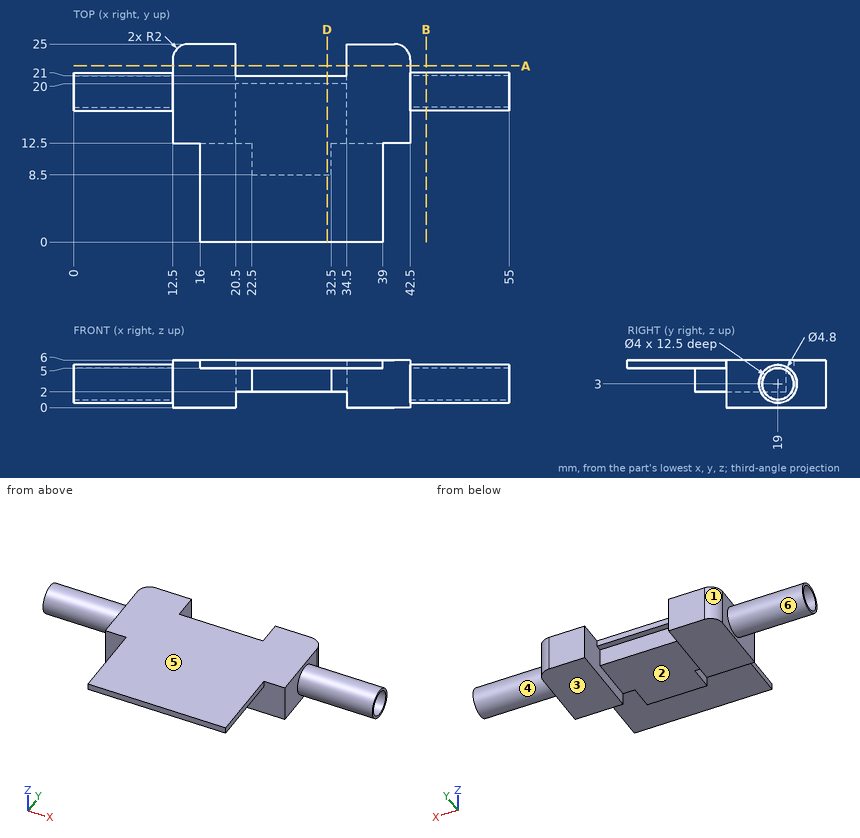
Verification items for this drawing (mm, ordinates from the low corner). A direction names the side the tool comes from. Round coordinates to 2 decimals unless told otherwise and drop trailing zeros. Loops run counter-clockwise (first coordinate to the right, second up) from the corner with the lowest first, then second, coordinate; pieces in that order, holes last. Notation, with made-up numbers: (33.25, 31.25) -> (60.25, 31.25) arc R21 cw to (60.25, 36.25) -> close; hole circle Ø7 at (-12, 40.5). An arc over 180 degrees is marked (long way). Write item = value, one per line. Start each with the question number.
1) Thickness scan on probe 1 along Y at (x, z) = (52.75, 3); probe 2 along Y at (x, z) = (22, 4.9); probe 3 along X at (y, z) = (15, 3.05). Record the ranges inside material, lowest first.
2) Release check for a two-part mould opening along X. For the marked faces 1, 2 and 3 record: released by +X, released by -X, zero draft, split by the parting line, or undercut.
3) Sectioned sample at B-B, the plane x = 44.5. Record the cut outline in (y, z).
4) Sectioned sample at A-A, the plane y = 22.25. Record the cut outline in (x, z), plus the area to 3 significant figures.
5) Set-up check for the marked faces 4, 5 and 6: record each of +Z, -Z, +X, -X, +Y, -Y from which the full face is reachable in a straight line by a thin tool's end or side.
6) Gauge pin test, flat ends, axial feed: pin 1 Ø2.5 at (y, z) = (19, 3) entering from +X; pin 2 Ø6 at (x, y) = (29.5, 6) entering from -Z; pin 3 Ø1.5 at (x, z) = (29.5, 3.5) entering from -Y. Record the tip position at first contact, or that the pin passes through.
7) Sectioned sample at D-D, the plane x = 32. Record the cut outline in (y, z).
Results are:
q1.probe_1 = 16.6 to 17, 21 to 21.4
q1.probe_2 = 12.5 to 20
q1.probe_3 = 12.5 to 42.5
q2.face_1 = released by -X
q2.face_2 = undercut
q2.face_3 = zero draft
q3.outline = circle Ø4.8 at (19, 3); hole circle Ø4 at (19, 3)
q4.outline = (12.5, 0) -> (20.5, 0) -> (20.5, 6) -> (12.5, 6) -> close; (34.5, 0) -> (42.5, 0) -> (42.5, 6) -> (34.5, 6) -> close
q4.area = 96.0 mm^2
q5.face_4 = +X
q5.face_5 = +Z, +X, -X, +Y, -Y
q5.face_6 = -X
q6.pin_1 = 42.5
q6.pin_2 = 2
q6.pin_3 = 8.5
q7.outline = (0, 5) -> (8.5, 5) -> (8.5, 2) -> (20, 2) -> (20, 5) -> (21, 5) -> (21, 6) -> (0, 6) -> close
